Model file for the job. Use its own axes, mm. A direction names the side the tool comes from. Round coordinates to 2 decimals unless told otherwise and drop trailing zeros. Write each loop counter-clockwise with the first axis right and the second up, starting at its lowest first coordinate (ties: lowest second). Pieces come first, ordered by that corner, then holes.
```python
from build123d import *

# Parameters (mm, degrees)
SKETCH1_W           = 156
SKETCH1_H           = 156
BOSS_EXTRUDE1_DEPTH = 202
FILLET1_R           = 23
SHELL1_T            = -3


with BuildPart() as part:
    # Sketch1 → Boss-Extrude1 (new body)
    with BuildSketch(Plane(origin=(0, 0, 0), x_dir=(1, 0, 0), z_dir=(0, 1, 0))):
        with Locations((8.769230769, -22.609756098)):
            Rectangle(SKETCH1_W, SKETCH1_H)
    extrude(amount=BOSS_EXTRUDE1_DEPTH)

    # Fillet1
    fillet1_edges = [part.edges().sort_by_distance(p)[0] for p in [
        (8.769230769, 0, -55.390243902),
        (86.769230769, 0, 22.609756098),
        (8.769230769, 0, 100.609756098),
        (-69.230769231, 0, 22.609756098),
        (-69.230769231, 101, -55.390243902),
        (86.769230769, 101, -55.390243902),
        (86.769230769, 101, 100.609756098),
        (-69.230769231, 101, 100.609756098),
    ]]
    fillet(fillet1_edges, radius=FILLET1_R)

    # Shell1
    shell1_openings = [part.faces().sort_by_distance(p)[0] for p in [
        (8.769230769, 202, 22.609756098),
    ]]
    offset(amount=SHELL1_T, openings=shell1_openings, kind=Kind.INTERSECTION)


solid = part.part
```
1) Cut at A-A on y = 117.5. List the corners of the cut face in (x, z).
2) Cut at C-C on x = -32. List the corners of the cut face in (y, z), and give its area (3 significant figures).
3) Cut at B-B on z = 19. List the corners of the cut face in (x, y).
4) Pull direction X, two halves, no side cores. Call faces 1 (the face through (-62.672, 6.916, 21.84)), 2 (the face through (9.539, 6.916, 94.051)), 3 (the face through (-66.231, 111, 23)): released by +X, released by -X, zero draft, split by the parting line, or undercut.
5) Flat gauge pins, fed straight in: pin 1 Ø10 at (x, z) = (-29.5, -17.5) entering from +Y; pin 2 Ø6 at (x, y) = (69.5, 29) entering from +Z. Where does each tip first touch, or does it go through?
6) Wall check: probe 1 along Z at (x, y) = (-44, 184.5); probe 2 along X at (y, z) = (60.5, 4.5); probe 3 along Y at (x, z) = (33.5, -21). Give the ranges that are in metal, low to high.
7) Which spindle directions (+Z, -Z, +X, -X, +Y, -Y) get a long thin tool onto all of the face, cutting with end or side? Do faces 4 (the face through (8, 0, 22)), 5 (the face through (8, 111, 97.61)). Say none if no direction does.
Result sheet:
1. outline: (-69.23, -32.39) arc R23 ccw to (-46.23, -55.39) - (63.77, -55.39) arc R23 ccw to (86.77, -32.39) - (86.77, 77.61) arc R23 ccw to (63.77, 100.61) - (-46.23, 100.61) arc R23 ccw to (-69.23, 77.61) - close; hole (-66.23, -32.39) arc R20 ccw to (-46.23, -52.39) - (63.77, -52.39) arc R20 ccw to (83.77, -32.39) - (83.77, 77.61) arc R20 ccw to (63.77, 97.61) - (-46.23, 97.61) arc R20 ccw to (-66.23, 77.61) - close
2. outline: (0, -32.39) arc R23 ccw to (23, -55.39) - (202, -55.39) - (202, -52.39) - (23, -52.39) arc R20 cw to (3, -32.39) - (3, 77.61) arc R20 cw to (23, 97.61) - (202, 97.61) - (202, 100.61) - (23, 100.61) arc R23 ccw to (0, 77.61) - close
2. area: 1,610 mm2
3. outline: (-69.23, 23) arc R23 ccw to (-46.23, 0) - (63.77, 0) arc R23 ccw to (86.77, 23) - (86.77, 202) - (83.77, 202) - (83.77, 23) arc R20 cw to (63.77, 3) - (-46.23, 3) arc R20 cw to (-66.23, 23) - (-66.23, 202) - (-69.23, 202) - close
4. face 1: released by -X
4. face 2: zero draft
4. face 3: undercut
5. pin 1: stops at y = 3
5. pin 2: stops at z = 100.45
6. probe 1: z = -55.39 to -52.39, 97.61 to 100.61
6. probe 2: x = -69.23 to -66.23, 83.77 to 86.77
6. probe 3: y = 0 to 3
7. face 4: +Z, -Z, +X, -X, -Y
7. face 5: +Y
